The figure shows three views and two pictorial views of one solid part (mm, origin at its lowest corner). Answer the questions. Give positions to 0.01 mm unless a question says otherwise; leave off trailing zeros. Loops run counter-clockwise (first coordinate to the right, second up) from the corner with the lowest first, then second, coordinate; pieces in that order, holes last. Notation, with made-up numbers: M -9,-37 L 44,-37 A36 ccw 44,1 Z; hole C -35,-14.75 d7. An arc over 180 degrees is marked long. One line per item, written item: value. Start each with the question number.
Q1. A cutting plane is placed at B-B, the plane y = 268.5. Determine the outline of the cut face in (x, z), and give its area (3 significant figures).
Q2. A cutting plane is placed at A-A, the plane x = 200. Determine the outline of the cut face in (y, z), and give its area (3 significant figures).
Q3. A cutting plane is placed at D-D, the plane z = 1.5. State how many separate pieces and enclosed holes the cut face has, and give its area (3 significant figures).
Q4. Flat-ended cylindrical pins translate along their axes: pin 1 (6.5 mm diameter, centred on x = 375, y = 200, fed in from +Z); pin 2 (3 mm diameter, centred on y = 150, z = 2, fed in from -X). Find the tip coordinate at first contact, or state that the pin passes through.
Q5. A cutting plane is placed at C-C, the plane x = 25. Determine the outline of the cut face in (y, z).
Q6. Consider L1, parallel to Y at x = 25, z = 1.45; L2, parallel to Y at x = 287.5, z = 1.8. Determine where each line is inside the solid, lowest interval first.
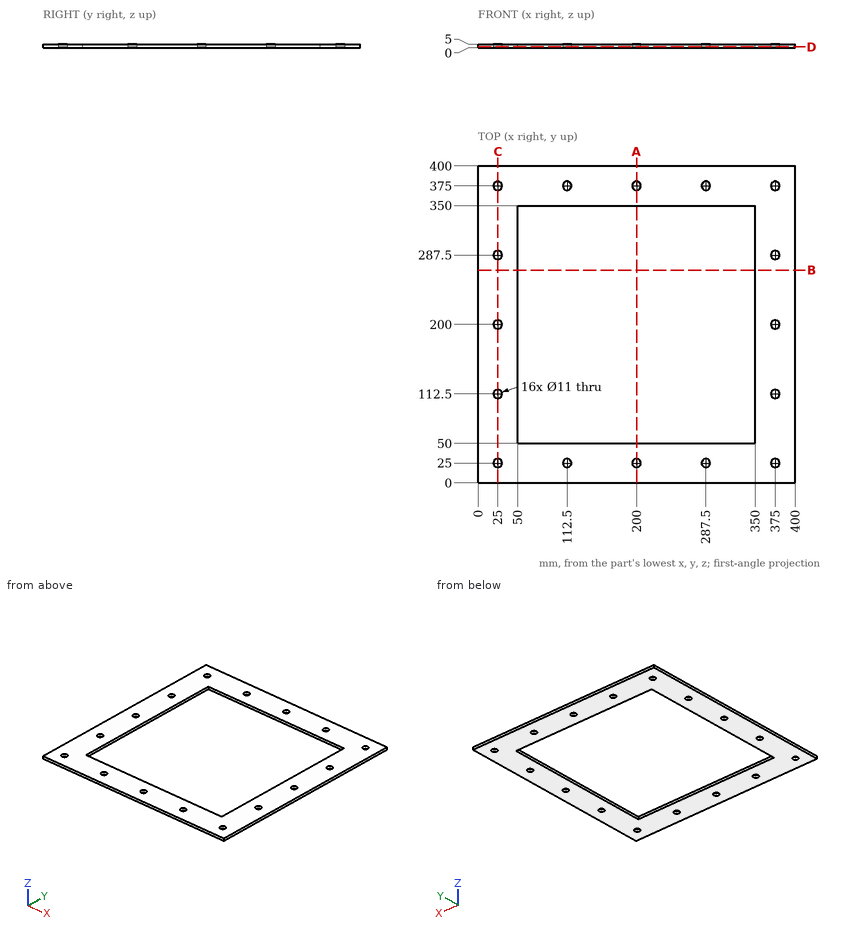
Answer block:
1. outline: M 0,0 L 50,0 L 50,5 L 0,5 Z; M 350,0 L 400,0 L 400,5 L 350,5 Z
1. area: 500 mm^2
2. outline: M 0,0 L 19.5,0 L 19.5,5 L 0,5 Z; M 30.5,0 L 50,0 L 50,5 L 30.5,5 Z; M 350,0 L 369.5,0 L 369.5,5 L 350,5 Z; M 380.5,0 L 400,0 L 400,5 L 380.5,5 Z
2. area: 390 mm^2
3. separate pieces: 1
3. enclosed holes: 17
3. area: 68,500 mm^2
4. pin 1: through
4. pin 2: x = 0
5. outline: M 0,0 L 19.5,0 L 19.5,5 L 0,5 Z; M 30.5,0 L 107,0 L 107,5 L 30.5,5 Z; M 118,0 L 194.5,0 L 194.5,5 L 118,5 Z; M 205.5,0 L 282,0 L 282,5 L 205.5,5 Z; M 293,0 L 369.5,0 L 369.5,5 L 293,5 Z; M 380.5,0 L 400,0 L 400,5 L 380.5,5 Z
6. L1: 0 to 19.5, 30.5 to 107, 118 to 194.5, 205.5 to 282, 293 to 369.5, 380.5 to 400
6. L2: 0 to 19.5, 30.5 to 50, 350 to 369.5, 380.5 to 400
